The listing builds one solid part. Answer for the finished solid, in the listing's coordinates (mm). Round coordinates to 2 decimals unless told otherwise and drop trailing zeros. Order: outer loops, then holes, each group sorted by start corner. A loop starts at its lowest first (then second) coordinate and runs counter-clockwise, first axis right, second up. Notation, with made-up numbers: M 55.25,58 L 97.25,58 A36 ccw 97.25,96 Z; hole C 29.25,16.5 d2. An arc over 180 degrees is marked long. Put each result on its own line as item: value. Start each with the question number.
1. Consider line 1 (Y direction, x = 497.5, z = 10.5); line 2 (X direction, y = -279, z = 7); line 3 (Y direction, x = 1197.5, z = 44). Determine where each line is inside the solid, lowest interval first.
2. The part is cut by section D-D (y = -259.5). Give the vertices of the cut face in (x, z), then the cut area to 3 significant figures.
3. Each of these flat-tipped pins is pushed along its axis until it touches: pin 1 Ø7.5 at (x, y) = (1205.5, 291) entering from +Z; pin 2 Ø7.5 at (x, y) = (16, -49.5) entering from -Z; pin 3 Ø12 at (y, z) = (68.5, 129.5) entering from +X; pin 4 Ø7.5 at (x, y) = (1252, 11.5) entering from +Z. Where does it stop, or does it pass through?
4. The part is cut by section C-C (y = 198.5). Give the vertices of the cut face in (x, z).
5. The part is cut by section B-B (x = 1016.5). Give the vertices of the cut face in (y, z), then the cut area to 3 significant figures.
6. The part is cut by section A-A (y = 4). Give the vertices of the cut face in (x, z).
from build123d import *

# Parameters (mm, degrees)
F0_W     = 25.4
F0_H     = 224.7411692651
F1_DEPTH = 25.4
F3_W     = 24.2299882889
F3_H     = 25.4
F4_DEPTH = 76.2
F5_W     = 25.4
F5_H     = 25.4
F6_DEPTH = 127
F7_W     = 25.4
F7_H     = 25.4
F8_DEPTH = 573.024


with BuildPart() as f1:
    # F0 (on Top) → F1 (new body)
    with BuildSketch(Plane.XY):
        Polygon((0, 304.8), (0, 0), (25.4, 0), (25.4, 33.1274457276), (25.4, 54.6588307349), (25.4, 279.4), (228.6, 279.4), (254, 279.4), (288.2145345211, 279.4), (313.6145345211, 279.4), (697.7127194405, 279.4), (723.1127194405, 279.4), (1194.9700117111, 279.4), (1237.9066371274, 54.6588307349), (1237.9066371274, 33.1274457276), (1237.9066371274, 0), (1263.3066371274, 0), (1263.3066371274, 54.6588307349), (1219.2, 304.8), align=None)
        Polygon((25.4, 54.6588307349), (25.4, 33.1274457276), (1237.9066371274, 33.1274457276), (1237.9066371274, 54.6588307349), (723.1127194405, 54.6588307349), (697.7127194405, 54.6588307349), (313.6145345211, 54.6588307349), (288.2145345211, 54.6588307349), (254, 54.6588307349), (228.6, 54.6588307349), align=None)
        with Locations((241.3, 167.0294153674)):
            Rectangle(F0_W, F0_H)
        with Locations((300.9145345211, 167.0294153674)):
            Rectangle(F0_W, F0_H)
        with Locations((710.4127194405, 167.0294153674)):
            Rectangle(F0_W, F0_H)
    extrude(amount=F1_DEPTH)

    # F2: F1 across plane


with BuildPart() as f1_1:
    add(f1.part)
    add(f1.part.mirror(Plane.XZ))

    # F3 (on face) → F4 (join)
    with BuildSketch(Plane.XY.offset(25.4)):
        with Locations((1207.0850058556, -292.1)):
            Rectangle(F3_W, F3_H)
        Polygon((1237.9066371274, -54.6588307349), (1263.3066371274, -54.6588307349), (1263.3066371274, -29.2588307349), (1237.9066371274, -29.2588307349), (1237.9066371274, -33.1274457276), align=None)
        Polygon((1237.9066371274, 29.2572733015), (1263.3066371274, 29.2572733015), (1263.3066371274, 54.6588307349), (1237.9066371274, 54.6588307349), (1237.9066371274, 33.1274457276), align=None)
        with Locations((1207.0850058556, 292.1)):
            Rectangle(F3_W, F3_H)
    extrude(amount=F4_DEPTH)

    # F5 (on face) → F6 (join)
    with BuildSketch(Plane.XY.offset(25.4)):
        with Locations((12.7, 292.1)):
            Rectangle(F5_W, F5_H)
        with Locations((12.7, -292.1)):
            Rectangle(F5_W, F5_H)
    extrude(amount=F6_DEPTH)

    # F7 (on face) → F8 (join)
    with BuildSketch(Plane.XZ.offset(-279.4)):
        with Locations((12.7, 139.7)):
            Rectangle(F7_W, F7_H)
    extrude(amount=F8_DEPTH)


solid = f1_1.part
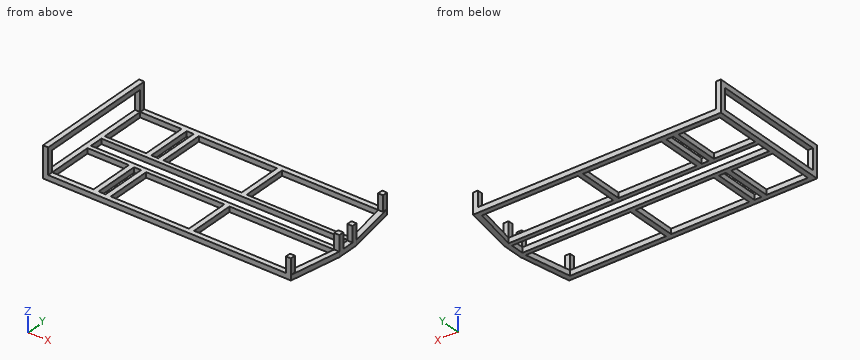
Resolved:
1. line 1: -304.8 to -279.4, -54.66 to -33.13, 33.13 to 54.66, 279.4 to 304.8
1. line 2: 0 to 25.4, 228.6 to 254, 288.21 to 313.61, 697.71 to 723.11, 1195.05 to 1223.75
1. line 3: -304.8 to -279.4, 279.4 to 304.8
2. outline: M 0,0 L 25.4,0 L 25.4,25.4 L 0,25.4 Z; M 0,127 L 25.4,127 L 25.4,152.4 L 0,152.4 Z; M 228.6,0 L 254,0 L 254,25.4 L 228.6,25.4 Z; M 288.21,0 L 313.61,0 L 313.61,25.4 L 288.21,25.4 Z; M 697.71,0 L 723.11,0 L 723.11,25.4 L 697.71,25.4 Z; M 1198.77,0 L 1227.19,0 L 1227.19,25.4 L 1198.77,25.4 Z
2. area: 3,950 mm2
3. pin 1: z = 101.6
3. pin 2: z = 0
3. pin 3: x = 25.4
3. pin 4: z = 25.4
4. outline: M 0,0 L 25.4,0 L 25.4,25.4 L 0,25.4 Z; M 0,127 L 25.4,127 L 25.4,152.4 L 0,152.4 Z; M 228.6,0 L 254,0 L 254,25.4 L 228.6,25.4 Z; M 288.21,0 L 313.61,0 L 313.61,25.4 L 288.21,25.4 Z; M 697.71,0 L 723.11,0 L 723.11,25.4 L 697.71,25.4 Z; M 1210.43,0 L 1237.94,0 L 1237.94,25.4 L 1210.43,25.4 Z
5. outline: M -304.8,0 L -279.4,0 L -279.4,25.4 L -304.8,25.4 Z; M -54.66,0 L -33.13,0 L -33.13,25.4 L -54.66,25.4 Z; M 33.13,0 L 54.66,0 L 54.66,25.4 L 33.13,25.4 Z; M 279.4,0 L 304.8,0 L 304.8,25.4 L 279.4,25.4 Z
5. area: 2,380 mm2
6. outline: M 0,0 L 25.4,0 L 25.4,25.4 L 0,25.4 Z; M 0,127 L 25.4,127 L 25.4,152.4 L 0,152.4 Z; M 1237.91,0 L 1263.31,0 L 1263.31,25.4 L 1237.91,25.4 Z
